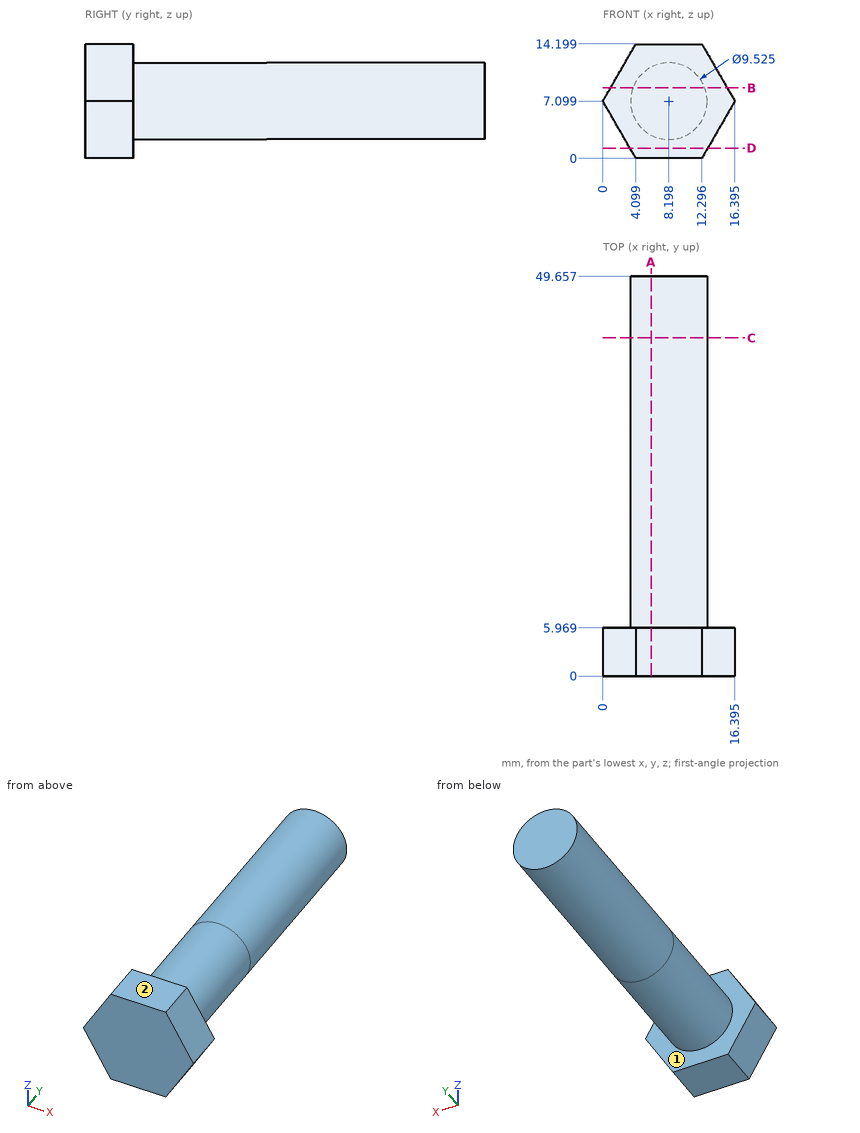
Input: dimensioned drawing with shaded views. Units: mm. Origin: part minimum x, y, z. A direction names the side the tool comes from. Give positions to 0.01 mm unless a question says otherwise; leave off trailing zeros. Write each loop counter-clockwise with the first axis right and the second up, starting at its lowest first coordinate (ties: lowest second). Pieces come first, ordered by that corner, then holes.
1. First-contact query: pin 1 (3 mm diameter, centred on x = 6.5, y = 13.5, fed in from +Z); pin 2 (5 mm diameter, centred on y = 40.5, z = 6, fed in from -X) (1 decimal); pin 3 (8 mm diameter, centred on x = 7.5, y = 41.5, fed in from -Z). Flat tips, straight axial feed; report the tip coordinate or a pass-through.
2. Section query B-B (z = 8.75). Return the cut outline in (x, y) (1 decimal).
3. Material intervals for line 1 along Y through (x, z) = (5.25, 12); line 2 along Z through (x, y) = (8, 12); line 3 along X through (y, z) = (29, 7.75) (1 decimal), sorted ascending.
4. Section query A-A (x = 6). Return the cut outline in (y, z) (1 decimal).
5. Access query for the marked faces 1 and 2. Directions: +Z, -Z, +X, -X, +Y, -Y. A direction counts if a zero-diameter tool reaches every point of the face in a straight line with its end or side. Return the directions, or none.
6. Section query D-D (z = 1.25). Return the cut outline in (x, y).
7. Section query C-C (y = 42). Return the cut outline in (x, z) (1 decimal).
Output values:
1. pin 1: stops at z = 11.86
1. pin 2: stops at x = 3.4
1. pin 3: stops at z = 2.34
2. outline: (1, 0) - (15.4, 0) - (15.4, 6) - (12.7, 6) - (12.7, 49.7) - (3.7, 49.7) - (3.7, 6) - (1, 6) - close
3. line 1: y = 0 to 5.97
3. line 2: z = 2.34 to 11.86
3. line 3: x = 3.5 to 12.9
4. outline: (0, 0) - (6, 0) - (6, 2.9) - (49.7, 2.9) - (49.7, 11.3) - (6, 11.3) - (6, 14.2) - (0, 14.2) - close
5. face 1: +Y
5. face 2: +Z, +X, -X, +Y, -Y
6. outline: (3.38, 0) - (13.02, 0) - (13.02, 5.97) - (3.38, 5.97) - close
7. outline: circle Ø9.5 at (8.2, 7.1)
